For this review, take the finished solid that the model builds, in its own axes (mm). A direction names the side the tool comes from. Coordinates: 2 decimals unless noted, no trailing zeros. Order: outer loops, then holes, each group sorted by start corner. A loop starts at its lowest first (then second) coordinate and runs counter-clockwise, first axis right, second up. Notation, with made-up numbers: (81, 42) - (103, 42) arc R7 cw to (103, 50) - close; hole circle Ø11 at (38, 6). An arc over 180 degrees is marked (long way). One line per item, written item: value. Start each with the question number.
(1) For faces 1 (the cylindrical face through (0.97, -18.89, -19.29)), 2 (the flat face through (0, -27, 11)), 3 (the cylindrical face through (4.437, 2.883, -1.5)), list the 3-axis set-ups (+Z, -Z, +X, -X, +Y, -Y) from which the entire face can be reached by the end or side of a thin tool; tool diameter is ignored.
(2) Consider section A-A on y = 0. Write out the cut boundary in (x, z) (3 decimals), then the cut area to 3 significant figures.
(3) Consider section D-D on y = -8. Write out the cut boundary in (x, z), then the cut area to 3 significant figures.
(4) Clearance check with flat-ended pins moving along their axes: pin 1 (1.2 mm diameter, centred on x = 0.5, z = -18, fed in from +Y); pin 2 (3 mm diameter, centred on x = 0.5, y = -13.5, fed in from +Z); pin 3 (2 mm diameter, centred on x = 1.5, z = -16.5, fed in from -Y). State where each tip first meets the part, or that it passes through.
(5) Mouldability with a two-part tool opening along X and no side actions: class faces 4 (the flat face through (2, -27, -11)), 5 (the flat face through (3, 0, 6)), 6 (the cylindrical face through (0.97, 18.89, 19.29)) as released by +X, released by -X, zero draft, split by the parting line, or undercut.
(6) To check wall thickness, follow line 1 along Y through (x, z) = (2.5, 0) (3 decimals); line 2 along Z through (x, y) = (2.75, 14); line 3 along Z through (x, y) = (5, 0) (3 decimals). State the ranges of each line that lie inside material, in increasing order.
(7) Consider section C-C on z = -21. Write out the cut boundary in (x, y), then the cut area to 3 significant figures.
Autodesk Inventor part; units mm, degrees
ref_plane "YZ Plane" through (0, 0, 0) normal (1, 0, 0) x (0, 1, 0)
ref_plane "XZ Plane" through (0, 0, 0) normal (0, 1, 0) x (-1, 0, 0)
ref_plane "XY Plane" through (0, 0, 0) normal (0, 0, 1) x (1, 0, 0)
sketch "Sketch1" plane through (0, 0, 0) normal (1, 0, 0) x (0, 1, 0)
  circle A0 centre (0, 0) radius 28.5
  dimension "d0" = 57
extrude "Extrusion1" add sketch "Sketch1" along normal blind 2
sketch "Sketch2" plane through (2, 0, 0) normal (1, 0, 0) x (0, 0, -1)
  circle A0 centre (0, 0) radius 30
  dimension "d3" = 60
extrude "Extrusion2" add sketch "Sketch2" along normal blind 1
sketch "Sketch3" plane through (0, 0, 0) normal (-1, 0, 0) x (0, 0, 1)
  circle A0 centre (0, 0) radius 30
  dimension "d6" = 60
extrude "Extrusion3" add sketch "Sketch3" along normal blind 1
sketch "Sketch4" plane through (-1, 0, 0) normal (-1, 0, 0) x (0, 0, 1)
  circle A0 centre (0, 0) radius 27
  dimension "d9" = 54
extrude "Extrusion4" cut sketch "Sketch4" against normal blind 10
sketch "Sketch5" plane through (-1, 0, 0) normal (-1, 0, 0) x (0, 0, 1)
  circle A0 centre (0, 0) radius 2.125
  circle A1 centre (0, 0) radius 3.25
  dimension "d12" = 4.25
  dimension "d13" = 6.5
extrude "Extrusion5" add sketch "Sketch5" against normal blind 4
sketch "Sketch6" plane through (-1, 0, 0) normal (-1, 0, 0) x (0, 0, 1)
  line L0 (-2.9572, 0) -> (-2.9572, 1) construction
  line L1 (-2.9572, 1) -> (-2.9572, -1) construction
  line L2 (-2.9572, 1) -> (-27.9528, 1)
  line L3 (-27.9528, 1) -> (-27.9528, -1)
  line L4 (-27.9528, -1) -> (-2.9572, -1)
  line L5 (-2.9572, -1) -> (-2.9572, 1)
  point P0 (0, 0)
  dimension "d16" = 1
  dimension "d17" = 2
extrude "Extrusion6" add sketch "Sketch6" against normal blind 4
pattern_circular "Circular Pattern1" count 4 over 360 about axis through (-1, 0, 0) along (1, 0, 0) of "Extrusion6"
sketch "Sketch7" plane through (3, 0, 0) normal (1, 0, 0) x (0, 0, -1)
  circle A0 centre (0, 0) radius 2.125
  circle A1 centre (0, 0) radius 3.25
extrude "Extrusion7" add sketch "Sketch7" along normal blind 5
properties part number "mtv_brakeWheel(61mm)_1-14"
Geometry check:
1. face 1: +X, -X
1. face 2: none
1. face 3: +X
2. outline: (-1, -30) - (0, -30) - (0, -28.5) - (2, -28.5) - (2, -30) - (3, -30) - (3, -3.25) - (8, -3.25) - (8, -2.125) - (-1, -2.125) - close; (-1, 2.125) - (8, 2.125) - (8, 3.25) - (3, 3.25) - (3, 30) - (2, 30) - (2, 28.5) - (0, 28.5) - (0, 30) - (-1, 30) - close
2. area: 228 mm^2
3. outline: (-1, -28.91) - (0, -28.91) - (0, -27.35) - (2, -27.35) - (2, -28.91) - (3, -28.91) - (3, -25.79) - (-1, -25.79) - close; (-1, -1) - (3, -1) - (3, 1) - (-1, 1) - close; (-1, 25.79) - (3, 25.79) - (3, 28.91) - (2, 28.91) - (2, 27.35) - (0, 27.35) - (0, 28.91) - (-1, 28.91) - close
3. area: 26.8 mm^2
4. pin 1: stops at y = 24.25
4. pin 2: stops at z = 27.46
4. pin 3: stops at y = -25.6
5. face 4: undercut
5. face 5: released by +X
5. face 6: zero draft
6. line 1: y = -30 to -2.125, 2.125 to 30
6. line 2: z = -26.53 to -23.09, -1 to 1, 23.09 to 26.53
6. line 3: z = -3.25 to -2.125, 2.125 to 3.25
7. outline: (-1, -21.42) - (0, -21.42) - (0, -19.27) - (2, -19.27) - (2, -21.42) - (3, -21.42) - (3, -16.97) - (-1, -16.97) - close; (-1, -1) - (3, -1) - (3, 1) - (-1, 1) - close; (-1, 16.97) - (3, 16.97) - (3, 21.42) - (2, 21.42) - (2, 19.27) - (0, 19.27) - (0, 21.42) - (-1, 21.42) - close
7. area: 35.0 mm^2
